Geometry: see drawing. Coordinates: mm, zero at the bounding-box minimum. Give positions to 0.01 mm unless a question says otherwise; leave off trailing zeros. Order: outer loops, then holes, each group sorted by start corner. A loop starts at its lowest first (then second) coordinate and runs counter-clockwise, first axis right, second up. Notation, with made-up numbers: (58, -19.5) - (117, -19.5) arc R22 cw to (117, -1.5) - close; hole circle Ø4 at (-2, 0). An arc over 180 degrees is marked (long way). One line per item, written item: value.
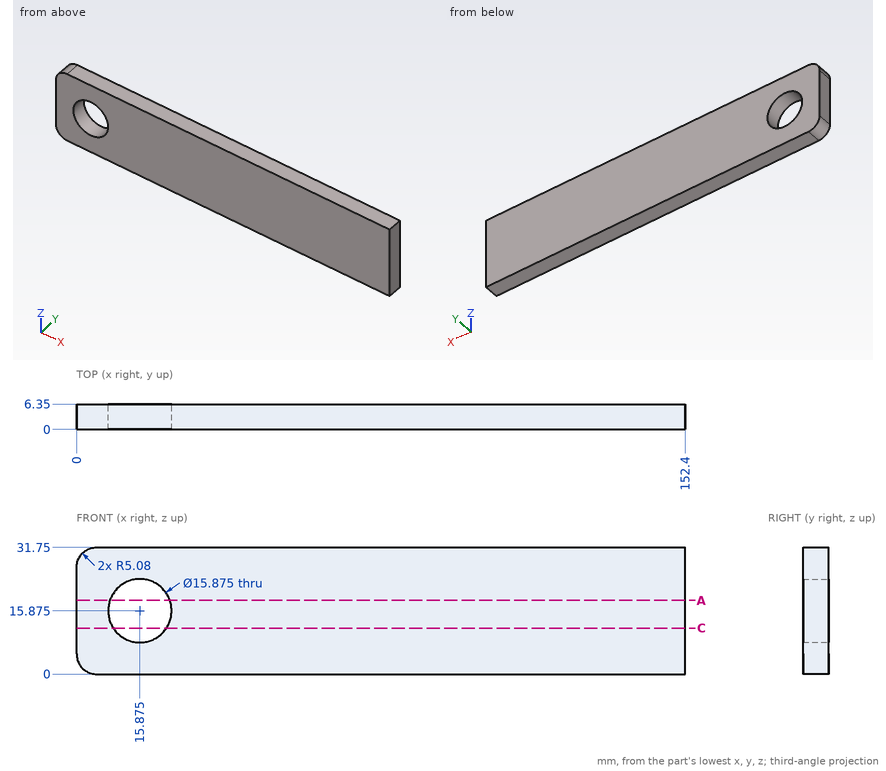
1) Section C-C, the plane z = 11.5. Return loops of the section in (x, y), then the cut area to 3 significant figures.
Answers below:
outline: (0, 0) - (9.25, 0) - (9.25, 6.35) - (0, 6.35) - close; (22.5, 0) - (152.4, 0) - (152.4, 6.35) - (22.5, 6.35) - close
area: 884 mm^2
2) Section A-A, the plane z = 18.5. Return loops of the section in (x, y).
Answers below:
outline: (0, 0) - (8.38, 0) - (8.38, 6.35) - (0, 6.35) - close; (23.37, 0) - (152.4, 0) - (152.4, 6.35) - (23.37, 6.35) - close
3) Material intervals for line 1 along X through (y, z) = (5.25, 14.5); line 2 along Z through (x, y) = (9.5, 3.75); line 3 along Z through (x, y) = (22, 5), sorted ascending.
Answers below:
line 1: 0 to 8.06, 23.69 to 152.4
line 2: 0 to 11.15, 20.6 to 31.75
line 3: 0 to 10.83, 20.92 to 31.75
